Part model, mm, in its own coordinate system. A direction names the side the tool comes from. Round coordinates to 2 decimals unless told otherwise and drop trailing zeros. Write each loop counter-clockwise with the first axis right and the second up, starting at its lowest first coordinate (ties: lowest second). Pieces come first, ordered by that corner, then holes. Notation, with made-up numbers: M 2,-32 L 46,-32 A11 ccw 46,-21 Z; hole C 33,5 d4. An arc over 180 degrees is marked long. Use a Markdown table: item, result. Add a question column.
1) Two-plate mould, pull along Z, no slides. Class faces 3 (the face through (-27.53, -592.33, -123.98)), 4 (the face through (50, -306, 125)), 5 (the face through (16, -340, 146.3)), 6 (the face through (-9.894, -214.647, 135.501)): released by +Z, released by -Z, zero draft, split by the parting line, or undercut.
2) Slice it at B-B on y = -504.5. Write the cut outline in (x, z).
3) Which spindle directions (+Z, -Z, +X, -X, +Y, -Y) get a long thin tool onto all of the face, cutting with end or side? Do faces 1 (the face through (-76, -605, 66)), 2 (the face through (-9, 0, -103)). Say none if no direction does.
4) Wall check: probe 1 along Y at (x, z) = (0, 135); probe 2 along Y at (x, z) = (-17, 117); probe 3 along Z at (x, y) = (70, -279.5). Give the ranges that are in metal, low to high.
5) Drop flat-ended pins along their axis: P1, Ø1, axis at x = -27.5, y = -167, coming from the +Z side; P2, Ø8, axis at y = -152, z = 91, coming from the -X side; P3, Ø4, axis at y = -239.5, z = 57, coming from the -X side. Give the stop position or say it passes through.
6) Slice it at A-A on z = 45.5. Write the cut outline in (x, y).
```python
from build123d import *

# Parameters (mm, degrees)
F0_R      = 102
F0_R_2    = 100
F1_DEPTH  = 580
F2_R      = 127
F2_R_2    = 102
F2_R_3    = 100
F3_DEPTH  = 25
F4_R      = 127
F4_R_2    = 102
F4_R_3    = 100
F5_DEPTH  = 25
F7_D      = 8.4
F9_R      = 52
F9_R_2    = 50
F10_REACH = 399.0792104868
F11_REACH = 393.4223562373
F9_R_3    = 76
F12_DEPTH = 21.3
F14_D     = 8.4
F14_DEPTH = 27
F14_TIP   = 2.5236145999


with BuildPart() as f1:
    # F0 (on Front) → F1 (new body)
    with BuildSketch(Plane.XZ):
        Circle(F0_R)
        Circle(F0_R_2, mode=Mode.SUBTRACT)
    extrude(amount=F1_DEPTH)

    # F2 (on face) → F3 (join)
    with BuildSketch(Plane.XZ.offset(580)):
        Circle(F2_R)
        Circle(F2_R_2, mode=Mode.SUBTRACT)
        Circle(F2_R_2)
        Circle(F2_R_3, mode=Mode.SUBTRACT)
    extrude(amount=F3_DEPTH)

    # F4 (on face) → F5 (join)
    with BuildSketch(Plane(origin=(0, 0, 0), x_dir=(-1, 0, 0), z_dir=(0, 1, 0))):
        Circle(F4_R)
        Circle(F4_R_2, mode=Mode.SUBTRACT)
        Circle(F4_R_2)
        Circle(F4_R_3, mode=Mode.SUBTRACT)
    extrude(amount=F5_DEPTH)

    # F7 (through all)
    with Locations(Plane(origin=(0, 25, 0), x_dir=(-1, 0, 0), z_dir=(0, 1, 0))):
        with Locations((0, 116), (30.0230092319, 112.0473958495), (58, 100.458946839), (82.0243866176, 82.0243866176), (100.458946839, 58), (112.0473958495, 30.0230092319), (116, 0), (112.0473958495, -30.0230092319), (100.458946839, -58), (82.0243866176, -82.0243866176), (58, -100.458946839), (30.0230092319, -112.0473958495), (0, -116), (-30.0230092319, -112.0473958495), (-58, -100.458946839), (-82.0243866176, -82.0243866176), (-100.458946839, -58), (-112.0473958495, -30.0230092319), (-116, 0), (-112.0473958495, 30.0230092319), (-100.458946839, 58), (-82.0243866176, 82.0243866176), (-58, 100.458946839), (-30.0230092319, 112.0473958495)):
            Hole(F7_D / 2)

    f10_end = f1.faces().sort_by_distance((-102, -290, 0))[0]
    # F9 (on offset) → F10 (join, up to a face of the model that its end follows)
    with BuildSketch(Plane.XY.offset(125)):
        with Locations((0, -290)):
            Circle(F9_R)
        with Locations((0, -290)):
            Circle(F9_R_2, mode=Mode.SUBTRACT)
    f10_long = extrude(amount=-F10_REACH, mode=Mode.PRIVATE)
    add(split(f10_long, bisect_by=f10_end, keep=Keep.ALL, mode=Mode.PRIVATE).solids().sort_by_distance((-50.5292178951, -290, 125))[0])

    f11_end = f1.faces().sort_by_distance((-100, -302.5, 0))[0]
    # F9 (on offset) → F11 (cut, up to a face of the model that its end follows)
    with BuildSketch(Plane.XY.offset(125)):
        with Locations((0, -290)):
            Circle(F9_R_2)
    f11_long = extrude(amount=-F11_REACH, mode=Mode.PRIVATE)
    add(split(f11_long, bisect_by=f11_end, keep=Keep.ALL, mode=Mode.PRIVATE).solids().sort_by_distance((0, -290, 125))[0], mode=Mode.SUBTRACT)

    # F9 (on offset) → F12 (join)
    with BuildSketch(Plane.XY.offset(125)):
        with Locations((0, -290)):
            Circle(F9_R_3)
        with Locations((0, -290)):
            Circle(F9_R, mode=Mode.SUBTRACT)
        with Locations((0, -290)):
            Circle(F9_R)
        with Locations((0, -290)):
            Circle(F9_R_2, mode=Mode.SUBTRACT)
    extrude(amount=F12_DEPTH)

    # F14
    with Locations(Plane.XY.offset(146.3)):
        with Locations((0, -224.85), (24.9318256186, -229.8092484569), (46.0680067943, -243.9319932057), (60.1907515431, -265.0681743814), (65.15, -290), (60.1907515431, -314.9318256186), (46.0680067943, -336.0680067943), (24.9318256186, -350.1907515431), (0, -355.15), (-24.9318256186, -350.1907515431), (-46.0680067943, -336.0680067943), (-60.1907515431, -314.9318256186), (-65.15, -290), (-60.1907515431, -265.0681743814), (-46.0680067943, -243.9319932057), (-24.9318256186, -229.8092484569)):
            Hole(F14_D / 2, depth=F14_DEPTH)
            with Locations((0, 0, -(F14_DEPTH + F14_TIP / 2))):  # 118° drill point
                Cone(0, F14_D / 2, F14_TIP, mode=Mode.SUBTRACT)


solid = f1.part
```
Entries:
| question | item | result |
|---|---|---|
| 1 | face 3 | split by the parting line |
| 1 | face 4 | undercut |
| 1 | face 5 | released by +Z |
| 1 | face 6 | zero draft |
| 2 | outline | C 0,0 d204; hole C 0,0 d200 |
| 3 | face 1 | +Z, -Z, +X, -X, -Y |
| 3 | face 2 | none |
| 4 | probe 1 | y = -366 to -359.35, -350.95 to -340, -240 to -229.05, -220.65 to -214 |
| 4 | probe 2 | y = -605 to -580, -339.14 to -337.02, -242.98 to -240.86, 0 to 25 |
| 4 | probe 3 | z = -74.19 to -71.41, 71.41 to 74.19, 125 to 146.3 |
| 5 | P1 | stops at z = 98.36 |
| 5 | P2 | stops at x = -53.24 |
| 5 | P3 | stops at x = -85.9 |
| 6 | outline | M -118.57,-605 L -89.05,-605 L -89.05,25 L -118.57,25 L -118.57,0 L -91.29,0 L -91.29,-580 L -118.57,-580 Z; M 89.05,-605 L 118.57,-605 L 118.57,-580 L 91.29,-580 L 91.29,0 L 118.57,0 L 118.57,25 L 89.05,25 Z |
